Can you work these out from the drawing? Everything is in mm from the part's minimum corner. Give positions to 0.01 mm unless a question says otherwise; leave off trailing zeros. Order: outer loops, then holes, each group sorted by start corner. A loop starts at its lowest first (then second) coordinate and runs counter-clockwise, first axis right, second up. Notation, with made-up numbers: (85, 62.5) - (120, 62.5) arc R15 cw to (120, 76.5) - close; hole circle Ø8 at (20, -27.5). An arc over 180 degrees is marked (long way). Write each question's results on one line, items separated by ' | '. Start each with the question number.
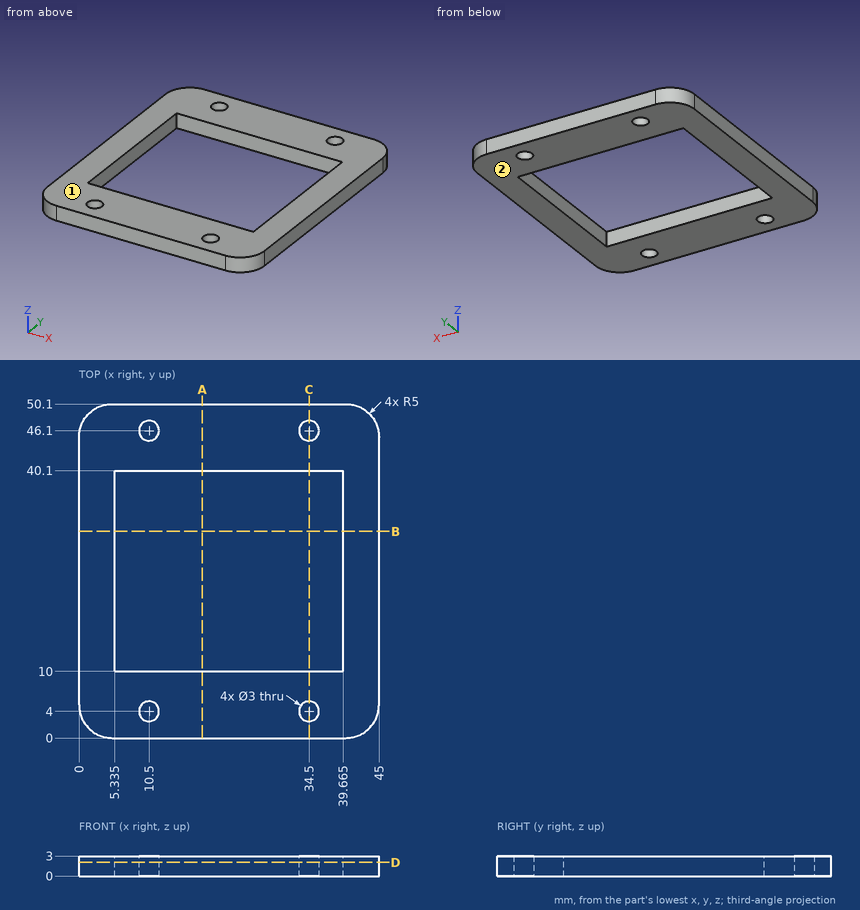
Q1. If we section it at C-C (x = 34.5): Please give me the cut outline in (y, z), plus the area to 3 significant figures.
Q2. If I drill on probe 1 along Y at (x, z) = (34.5, 1); probe 2 along X at (y, z) = (16, 0.5) (1 decimal); probe 3 along Y at (x, z) = (38.5, 2.8), over which ranges is the centre line in solid material (lowest first)? Write a range as from..to.
Q3. If we section it at D-D (z = 2.05): Please give me the cut outline in (x, y) (1 decimal), plus the area to 3 significant figures.
Q4. Thinking about a two-plate mould opening in Z: for the marked faces 1 and 2, which applies, released by +Z, released by -Z, zero draft, split by the parting line, or undercut?
Q5. If we section it at A-A (x = 18.5): Please give me the cut outline in (y, z), plus the area to 3 significant figures.
Q6. If we section it at B-B (y = 31): Please give me the cut outline in (x, z) (1 decimal), plus the area to 3 significant figures.
Findings below:
1) outline: (0, 0) - (2.5, 0) - (2.5, 3) - (0, 3) - close; (5.5, 0) - (10, 0) - (10, 3) - (5.5, 3) - close; (40.1, 0) - (44.6, 0) - (44.6, 3) - (40.1, 3) - close; (47.6, 0) - (50.1, 0) - (50.1, 3) - (47.6, 3) - close | area: 42.0 mm2
2) probe 1: y = 0..2.5, 5.5..10, 40.1..44.6, 47.6..50.1 | probe 2: x = 0..5.3, 39.7..45 | probe 3: y = 0..10, 40.1..50.1
3) outline: (0, 5) arc R5 ccw to (5, 0) - (40, 0) arc R5 ccw to (45, 5) - (45, 45.1) arc R5 ccw to (40, 50.1) - (5, 50.1) arc R5 ccw to (0, 45.1) - close; hole (5.3, 10) - (39.7, 10) - (39.7, 40.1) - (5.3, 40.1) - close; hole circle Ø3 at (10.5, 4); hole circle Ø3 at (10.5, 46.1); hole circle Ø3 at (34.5, 4); hole circle Ø3 at (34.5, 46.1) | area: 1,170 mm2
4) face 1: released by +Z | face 2: released by -Z
5) outline: (0, 0) - (10, 0) - (10, 3) - (0, 3) - close; (40.1, 0) - (50.1, 0) - (50.1, 3) - (40.1, 3) - close | area: 60.0 mm2
6) outline: (0, 0) - (5.3, 0) - (5.3, 3) - (0, 3) - close; (39.7, 0) - (45, 0) - (45, 3) - (39.7, 3) - close | area: 32.0 mm2
